Verification items for the finished model (mm, model axes). A direction names the side the tool comes from. Give positions to 0.01 mm unless a question says otherwise; leave off trailing zeros. Order: outer loops, then holes, each group sorted by start corner. A loop starts at its lowest first (then second) coordinate and runs counter-clockwise, first axis right, second up. Notation, with made-up numbers: (70.25, 68) - (112.25, 68) arc R22 cw to (112.25, 89) - close; hole circle Ø5 at (16, 35.5). An arc over 180 degrees is marked (long way). Answer as a JSON object with one key per item and string values. Group by question number.
(1) Section check C-C (y = 57.2). Record the boundary of the cut face in (x, z), then the cut area to 3 significant figures.
(2) Access from +Z, -Z, +X, -X, +Y, -Y to the whole of each face (thin tool, end or side, straight path). Record for faces 1 (the face through (30, 46, -12.5)), 2 (the face through (27.479, 61.416, 2.688)), 3 (the face through (26, 53, 3)), 4 (the face through (35.7, 39.7, 0.3)).
(3) Section check A-A (z = 0). Record the boundary of the cut face in (x, y), then the cut area to 3 significant figures.
(4) Thickness scan on line 1 (Y direction, x = 28, z = 0); line 2 (Z direction, x = -27, y = 57); line 3 (X direction, y = 23, z = -16). Record the ranges inside material, lowest first.
(5) Section check B-B (y = 32). Record the boundary of the cut face in (x, z).
(6) Mould release check, pull along Y, two halves, no side actions. Record for faces 5 (the face through (-35.1, 12.7, 7.8)), 6 (the face through (-30, 71, 0)), 7 (the face through (39.05, 3.94, 8.67)): +Y half, -Y half, draft (parallel to the pull), parting line (faces both ways), or undercut.
(7) Depth check by flat-ended pin: pin 1 Ø1 at (x, z) = (-24.5, 28) entering from +Y; pin 2 Ø3 at (y, z) = (7.5, -31) entering from -X; pin 3 Ø4 at (x, y) = (-29.5, 48.5) entering from -Z. Enter the tip coordinate at first touch or a pass-through.
```python
from build123d import *

# Parameters (mm, degrees)
SKETCH_1_R               = 40
EXTRUDE_1_DEPTH          = 13
SKETCH_3_R               = 35.699999999999996
EXTRUDE_2_DEPTH          = 58
CUT_EXTRUDE_1_DEPTH      = 58
CUT_EXTRUDE_1_DEPTH_BACK = 58
CUT_EXTRUDE_2_DEPTH      = 58
CUT_EXTRUDE_2_DEPTH_BACK = 58
SKETCH_6_R               = 4.999999999999999
CUT_EXTRUDE_3_DEPTH      = 3


with BuildPart() as part:
    # Sketch 1 → Extrude 1 (new body)
    with BuildSketch(Plane(origin=(0, 0, 0), x_dir=(1, 0, 0), z_dir=(0, 1, 0))):
        with Locations(Location((0, 0, 0), (0, 0, 90))):
            Circle(SKETCH_1_R)
    extrude(amount=EXTRUDE_1_DEPTH)

    # Sketch 2 → Cut-Revolve 1 (revolve, cut)
    with BuildSketch(Plane.XY, mode=Mode.PRIVATE) as cut_revolve_1_sk:
        Polygon((-35.7, 13.000000000000014), (-39.99999999999999, 8), (-39.99999999999999, 13), align=None)
    revolve(cut_revolve_1_sk.sketch.rotate(Axis((0, 13, 0), (0, -1, 0)), 90), axis=Axis((0, 13, 0), (0, -1, 0)), mode=Mode.SUBTRACT)

    # Sketch 3 → Extrude 2 (add)
    with BuildSketch(Plane(origin=(0, 13, 0), x_dir=(1, 0, 0), z_dir=(0, 1, 0))):
        with Locations(Location((0, 0, 0), (0, 0, 90))):
            Circle(SKETCH_3_R)
    extrude(amount=EXTRUDE_2_DEPTH)

    # Sketch 4 → Cut-Extrude 1 (cut, two sides: drawn at the far end of the back side and taken through both)
    with BuildSketch(Plane(origin=(0, 0, 0), x_dir=(0, 0, -1), z_dir=(1, 0, 0)).offset(-CUT_EXTRUDE_1_DEPTH_BACK)):
        with BuildLine():
            ThreePointArc((-35.7, 13.00000000000001), (-19.374333005026, 23.084447347021545), (-12.5, 41.00000000000001))
            Line((-12.5, 41.00000000000001), (-12.5, 51.35277843758252))
            ThreePointArc((-12.500000000000005, 51.352778437582536), (-11.64327397172637, 64.60771025481691), (-4.4e-16, 71.00000000000003))
            Line((0, 71.00000000000001), (-35.699999999999996, 71.00000000000001))
            Line((-35.699999999999996, 71.00000000000001), (-35.7, 13.000000000000014))
        make_face()
        with BuildLine():
            Line((35.699999999999996, 71.00000000000001), (0, 71.00000000000001))
            ThreePointArc((-4.4e-16, 71.00000000000003), (11.64327397172637, 64.60771025481691), (12.5, 51.35277843758252))
            Line((12.5, 51.35277843758252), (12.5, 41.00000000000001))
            ThreePointArc((12.5, 41.00000000000001), (19.374333005026003, 23.084447347021552), (35.7, 13.000000000000014))
            Line((35.7, 13.000000000000014), (35.699999999999996, 71.00000000000001))
        make_face()
    extrude(amount=CUT_EXTRUDE_1_DEPTH + CUT_EXTRUDE_1_DEPTH_BACK, mode=Mode.SUBTRACT)

    # Sketch 5 → Cut-Extrude 2 (cut, two sides: drawn at the far end of the back side and taken through both)
    with BuildSketch(Plane.XY.offset(-CUT_EXTRUDE_2_DEPTH_BACK)):
        Polygon((-26, 41.00000000000001), (-25.999999999999996, 71.00000000000001), (26, 71.00000000000001), (26, 41.00000000000001), align=None)
        with BuildLine():
            Line((-26, 41.00000000000001), (26, 41.00000000000001))
            ThreePointArc((26, 41.00000000000001), (-4.78e-15, 15.000000000000007), (-26, 41.00000000000001))
        make_face()
    extrude(amount=CUT_EXTRUDE_2_DEPTH + CUT_EXTRUDE_2_DEPTH_BACK, mode=Mode.SUBTRACT)

    # Sketch 6 → Cut-Extrude 3 (cut)
    with BuildSketch(Plane.ZY.offset(-26)):
        with Locations((0, 57.20000000000001)):
            Circle(SKETCH_6_R)
    cut_extrude_3 = extrude(amount=-CUT_EXTRUDE_3_DEPTH, mode=Mode.SUBTRACT)

    # Mirror 1: Cut-Extrude 3 across plane
    add(cut_extrude_3.mirror(Plane(origin=(0, 0, 0), x_dir=(0, 0, 1), z_dir=(1, 0, 0))), mode=Mode.SUBTRACT)


solid = part.part
```
Solutions:
{
 "1": {"outline": "(-32.92, -13.8) - (-26, -13.8) - (-26, -5) - (-29, -5) - (-29, 5) - (-26, 5) - (-26, 13.8) - (-32.92, 13.8) arc R35.7 ccw to start; (26, -13.8) - (32.92, -13.8) arc R35.7 ccw to (32.92, 13.8) - (26, 13.8) - (26, 5) - (29, 5) - (29, -5) - (26, -5) - close", "area": "425 mm2"},
 "2": {"face 1": "-Z, +X, -X", "face 2": "none", "face 3": "+Z, -Z, +Y", "face 4": "+X, +Y"},
 "3": {"outline": "(-40, 0) - (40, 0) - (40, 8) - (35.7, 13) - (35.7, 71) - (26, 71) - (26, 62.2) - (29, 62.2) - (29, 52.2) - (26, 52.2) - (26, 41) arc R26 cw to (-26, 41) - (-26, 52.2) - (-29, 52.2) - (-29, 62.2) - (-26, 62.2) - (-26, 71) - (-35.7, 71) - (-35.7, 13) - (-40, 8) - close", "area": "2,480 mm2"},
 "4": {"line 1": "y = 0 to 52.2, 62.2 to 71", "line 2": "z = -13.8 to -5, 5 to 13.8", "line 3": "x = -31.91 to -18.76, 18.76 to 31.91"},
 "5": {"outline": "(-32.72, -14.27) - (-24.39, -14.27) - (-24.39, 14.27) - (-32.72, 14.27) arc R35.7 ccw to start; (24.39, -14.27) - (32.72, -14.27) arc R35.7 ccw to (32.72, 14.27) - (24.39, 14.27) - close"},
 "6": {"face 5": "+Y half", "face 6": "undercut", "face 7": "draft"},
 "7": {"pin 1": "stops at y = 11.83", "pin 2": "stops at x = -27.01", "pin 3": "stops at z = -12.5"}
}
